Design review of the part built by this model. Coordinates are the model's own, in mm. Face numbers are marked on the shaded views. Coordinates: 2 decimals unless noted, no trailing zeros. Loops run counter-clockwise (first coordinate to the right, second up) from the corner with the lowest first, then second, coordinate; pieces in that order, holes last.
Q1. For P1, Ø6, axis at y = 10, z = 154.5, coming from the +X side; P2, Ø6, axis at x = 1, z = 212.5, coming from the -Y side (3 decimals); P3, Ø4, axis at y = 13, z = 249.5, coming from the +X side; P4, Ø1.5, axis at y = 13, z = 525.5, coming from the +X side, all flat-tipped, find the tip position at first contact; note any pin that passes through.
Q2. Draft analysis for pull direction X (two halves, no side actions). For the marked faces 1 and 2, state which applies: released by +X, released by -X, zero draft, split by the parting line, or undercut.
Q3. Add section A-A on x = 114. Give the boundary of the cut face in (y, z) (3 decimals).
Q4. Wall thickness on probe 1 along Z at (x, y) = (102, 4.25); probe 2 along Z at (x, y) = (-155, 7.75); probe 3 along X at (y, z) = (16, 406) (3 decimals): over which ranges is each line inside the solid? List them lowest first.
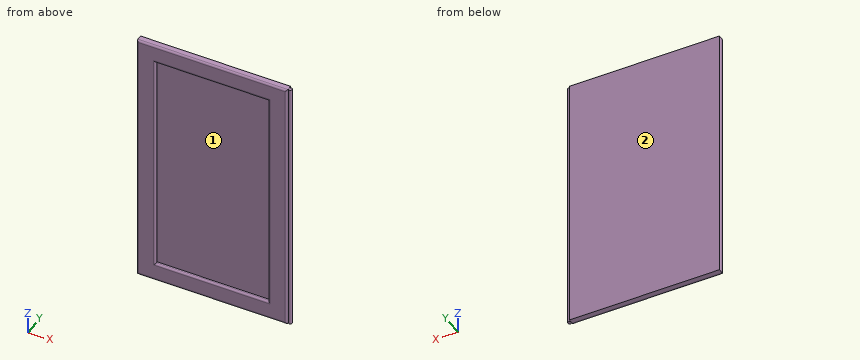
```python
from build123d import *

# Parameters (mm, degrees)
F0_W     = 412.75
F0_H     = 730.25
F1_DEPTH = 19.05
F3_DEPTH = 730.25
F4_W     = 311.15
F4_H     = 628.65
F5_DEPTH = 9.525
F6_R     = 5.08


with BuildPart() as f1:
    # F0 (on Front) → F1 (new body)
    with BuildSketch(Plane.XZ):
        with Locations((0, 365.125)):
            Rectangle(F0_W, F0_H)
    extrude(amount=-F1_DEPTH)

    # F2 (on Top) → F3 (join, through all)
    with BuildSketch(Plane.XY):
        with BuildLine():
            Line((204.7875, 7.9375), (206.6473719395, 7.9375))
            ThreePointArc((206.6473719395, 7.9375), (215.9, 9.525), (206.6473719395, 11.1125))
            Line((206.6473719395, 11.1125), (204.7875, 11.1125))
            Line((204.7875, 11.1125), (204.7875, 7.9375))
        make_face()
    extrude(amount=F3_DEPTH)

    # F4 (on Front) → F5 (cut)
    with BuildSketch(Plane.XZ):
        with Locations((0, 365.125)):
            Rectangle(F4_W, F4_H)
    extrude(amount=-F5_DEPTH, mode=Mode.SUBTRACT)

    # F6
    f6_edges = [f1.edges().sort_by_distance(p)[0] for p in [
        (-206.375, 0, 365.125),
        (0, 0, 730.25),
        (0, 0, 0),
        (206.375, 0, 365.125),
        (155.575, 0, 365.125),
        (0, 0, 679.45),
        (-155.575, 0, 365.125),
        (0, 0, 50.8),
    ]]
    fillet(f6_edges, radius=F6_R)


solid = f1.part
```
Entries:
1. P1: stops at x = 215.9
1. P2: stops at y = 9.525
1. P3: stops at x = 215.67
1. P4: stops at x = 215.04
2. face 1: undercut
2. face 2: zero draft
3. outline: (0, 5.08) arc R5.08 ccw to (5.08, 0) - (19.05, 0) - (19.05, 730.25) - (5.08, 730.25) arc R5.08 ccw to (0, 725.17) - (0, 684.53) arc R5.08 ccw to (5.08, 679.45) - (9.525, 679.45) - (9.525, 50.8) - (5.08, 50.8) arc R5.08 ccw to (0, 45.72) - close
4. probe 1: z = 0.07 to 50.73, 679.52 to 730.18
4. probe 2: z = 0 to 50.8, 679.45 to 730.25
4. probe 3: x = -206.375 to 206.375
